Drawing for the job (mm, zero at the part's lowest x, y, z). Give positions to 0.01 mm unless a question says otherwise; leave off trailing zeros. Order: outer loops, then holes, each group sorted by start corner. A loop starts at its lowest first (then second) coordinate and runs counter-clockwise, first axis right, second up. Notation, with made-up numbers: M -1,61 L 29,61 A26 ccw 29,78 Z; hole C 38,23 d4. An arc over 180 degrees is marked long. One line per item, written item: value.
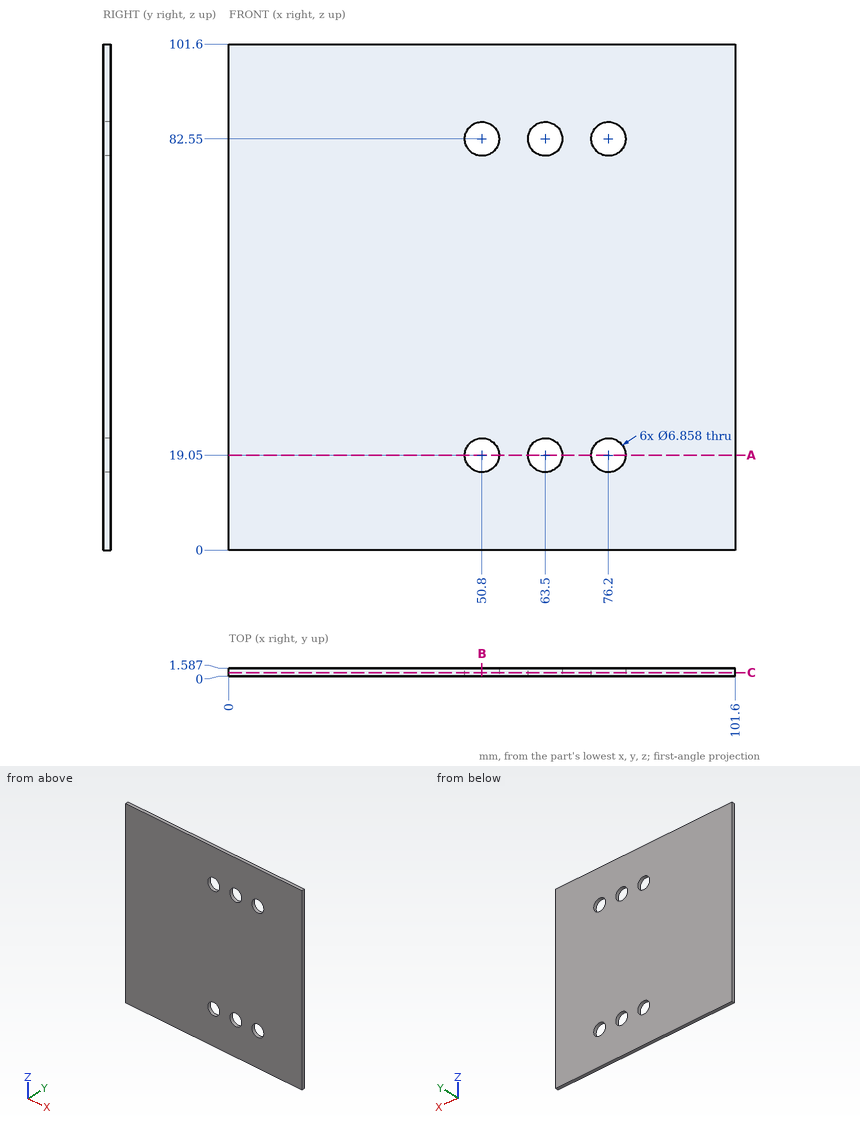
1) Saw through at B-B, the plane x = 50.8. Write the cut outline in (y, z).
Check values:
outline: M 0,0 L 1.59,0 L 1.59,15.62 L 0,15.62 Z; M 0,22.48 L 1.59,22.48 L 1.59,79.12 L 0,79.12 Z; M 0,85.98 L 1.59,85.98 L 1.59,101.6 L 0,101.6 Z
2) Saw through at A-A, the plane z = 19.05. Write the cut outline in (x, y).
Check values:
outline: M 0,0 L 47.37,0 L 47.37,1.59 L 0,1.59 Z; M 54.23,0 L 60.07,0 L 60.07,1.59 L 54.23,1.59 Z; M 66.93,0 L 72.77,0 L 72.77,1.59 L 66.93,1.59 Z; M 79.63,0 L 101.6,0 L 101.6,1.59 L 79.63,1.59 Z
3) Saw through at C-C, the plane y = 0.7. Write the cut outline in (x, z), then the cut area to 3 significant figures.
Check values:
outline: M 0,0 L 101.6,0 L 101.6,101.6 L 0,101.6 Z; hole C 50.8,19.05 d6.86; hole C 50.8,82.55 d6.86; hole C 63.5,19.05 d6.86; hole C 63.5,82.55 d6.86; hole C 76.2,19.05 d6.86; hole C 76.2,82.55 d6.86
area: 10,100 mm^2
4) Drill centre lines: probe 1 along Z at (x, y) = (76.2, 0.9); probe 2 along X at (y, z) = (1.45, 81); probe 3 along X at (y, z) = (0.85, 85). Where is each one in solid material? Low to high. Write a range as from..to.
Check values:
probe 1: 0..15.62, 22.48..79.12, 85.98..101.6
probe 2: 0..47.74, 53.86..60.44, 66.56..73.14, 79.26..101.6
probe 3: 0..48.4, 53.2..61.1, 65.9..73.8, 78.6..101.6
